from build123d import *

# Parameters (mm, degrees)
SKETCH1_R           = 4.1
BOSS_EXTRUDE1_DEPTH = 4.5
SKETCH2_W           = 4
SKETCH2_H           = 26
BOSS_EXTRUDE2_DEPTH = 58
SKETCH3_W           = 5
SKETCH3_H           = 26
BOSS_EXTRUDE3_DEPTH = 38
CUT_EXTRUDE1_START  = -5
CUT_EXTRUDE1_DEPTH  = 3
SKETCH6_R           = 4.2
CUT_EXTRUDE2_DEPTH  = 10
FILLET1_R           = 12
CUT_EXTRUDE4_DEPTH  = 74
SKETCH8_R           = 1.599994812
SKETCH8_R_2         = 1.6
SKETCH8_R_3         = 1.599991008
CUT_EXTRUDE5_DEPTH  = 8.5
CUT_EXTRUDE6_DEPTH  = 2
SKETCH10_W          = 7
SKETCH10_H          = 2.5
CUT_EXTRUDE7_DEPTH  = 114


with BuildPart() as part:
    # Sketch1 → Boss-Extrude1 (new body)
    with BuildSketch(Plane.XY):
        with BuildLine():
            Line((58.8, 13), (93.910980652, 13))
            Line((93.910980652, 13), (93.910980652, -13))
            Line((93.910980652, -13), (58.8, -13))
            ThreePointArc((58.8, -13), (45.8, 0), (58.8, 13))
        make_face()
        with Locations((58.8, 0)):
            Circle(SKETCH1_R, mode=Mode.SUBTRACT)
    extrude(amount=BOSS_EXTRUDE1_DEPTH)

    # Sketch2 → Boss-Extrude2 (add)
    with BuildSketch(Plane.XY.offset(4.5)):
        with Locations((91.910980652, 0)):
            Rectangle(SKETCH2_W, SKETCH2_H)
    extrude(amount=BOSS_EXTRUDE2_DEPTH)

    # Sketch3 → Boss-Extrude3 (add)
    with BuildSketch(Plane.ZY.offset(-89.910980652)):
        with Locations((60, 0)):
            Rectangle(SKETCH3_W, SKETCH3_H)
    extrude(amount=BOSS_EXTRUDE3_DEPTH)

    # Sketch5 → Cut-Extrude1 (cut)
    with BuildSketch(Plane.XY.offset(62.5).offset(CUT_EXTRUDE1_START)):
        with BuildLine():
            Line((75.8, 1.8), (59.925839282, 3.994369276))
            ThreePointArc((59.925839282, 3.994369276), (54.65, 6.2252e-05), (59.925719446, -3.99440305))
            Line((59.925719446, -3.99440305), (75.8, -1.799997977))
            ThreePointArc((75.8, -1.799997977), (77.599998989, 1.011e-06), (75.8, 1.8))
        make_face()
    extrude(amount=CUT_EXTRUDE1_DEPTH, mode=Mode.SUBTRACT)

    # Sketch6 → Cut-Extrude2 (cut)
    with BuildSketch(Plane.XY.offset(62.5)):
        with Locations((58.8, 0)):
            Circle(SKETCH6_R)
    extrude(amount=-CUT_EXTRUDE2_DEPTH, mode=Mode.SUBTRACT)

    # Fillet1
    fillet1_edges = [part.edges().sort_by_distance(p)[0] for p in [
        (51.910980652, 13, 60),
        (51.910980652, -13, 60),
    ]]
    fillet(fillet1_edges, radius=FILLET1_R)

    # Sketch7 → Cut-Extrude4 (cut)
    with BuildSketch(Plane(origin=(0, 0, 0), x_dir=(-1, 0, 0), z_dir=(0, 0, -1))):
        Polygon((-56.262443614, -3.220373827), (-56.262443614, 3.220373827), (-53.042069787, 0), align=None)
    extrude(amount=-CUT_EXTRUDE4_DEPTH, mode=Mode.SUBTRACT)

    # Sketch8 → Cut-Extrude5 (cut)
    with BuildSketch(Plane(origin=(93.910980652, 0, 0), x_dir=(0, 0, -1), z_dir=(1, 0, 0))):
        with Locations((-53.458782271, -8.985219923)):
            Circle(SKETCH8_R)
        with Locations((-53.458782271, 9)):
            Circle(SKETCH8_R_2)
        with Locations((-33.458782271, 9)):
            Circle(SKETCH8_R_2)
        with Locations((-33.458782271, -8.985219923)):
            Circle(SKETCH8_R_3)
    extrude(amount=-CUT_EXTRUDE5_DEPTH, mode=Mode.SUBTRACT)

    # Sketch9 → Cut-Extrude6 (cut)
    with BuildSketch(Plane.ZY.offset(-89.910980652)):
        Polygon((30.587828745, -7.37661001), (30.630208458, -10.667233653), (33.501161984, -12.275843566), (36.329735796, -10.593829837), (36.287356083, -7.303206194), (33.416402558, -5.69459628), align=None)
        Polygon((30.584160019, 10.602044603), (30.63405982, 7.311526406), (33.508682072, 5.709481802), (36.333404522, 7.397955397), (36.283504721, 10.688473594), (33.408882469, 12.290518198), align=None)
        Polygon((50.589182836, -7.374195689), (50.62879464, -10.664853815), (53.498394075, -12.27587805), (56.328381705, -10.596244158), (56.288769901, -7.305586031), (53.419170466, -5.694561797), align=None)
        Polygon((50.692796157, 7.216934993), (53.619968806, 5.713053256), (56.38595492, 7.496118262), (56.224768384, 10.783065007), (53.297595735, 12.286946744), (50.531609621, 10.503881738), align=None)
    extrude(amount=-CUT_EXTRUDE6_DEPTH, mode=Mode.SUBTRACT)

    # Sketch10 → Cut-Extrude7 (cut)
    with BuildSketch(Plane(origin=(0, 0, 0), x_dir=(-1, 0, 0), z_dir=(0, 0, -1))):
        with Locations((-84.62488512, 9.639193317)):
            Rectangle(SKETCH10_W, SKETCH10_H)
    extrude(amount=-CUT_EXTRUDE7_DEPTH, mode=Mode.SUBTRACT)


solid = part.part
Build history of the part. All positions in model axes, mm. A direction names the side the tool comes from. Give positions to 0.01 mm unless a question says otherwise; leave off trailing zeros. Loops run counter-clockwise (first coordinate to the right, second up) from the corner with the lowest first, then second, coordinate; pieces in that order, holes last. Notation, with made-up numbers: (-26, -39) - (4, -39) arc R23 cw to (4, -31) - close; hole circle Ø1 at (78, 24.25). An arc over 180 degrees is marked (long way). Write item = value, one per line. Start each with the question number.
1) Probe probe 1 along Z at (x, y) = (75.5, 6.25); probe 2 along X at (y, z) = (2.5, 55.5); probe 3 along Z at (x, y) = (52.5, -10). List the from-to ranges inside material, lowest first. Write a range as from..to.
2) Drop flat-ended pins along their axis: pin 1 Ø6.5 at (y, z) = (-7.5, 32.5) entering from -X; pin 2 Ø3 at (y, z) = (9, 53.46) entering from +X; pin 3 Ø3.5 at (y, z) = (-8.99, 53.46) entering from -X. Give the stop position or say it passes through.
3) Pull direction Y, two halves, no side cores. Call faces 4 (the cylindrical face through (55.52, -9.58, 60.04)), 5 (the flat face through (68, 0, 4.5)), 6 (the cylindrical face through (55.84, -2.98, 60.59)), 7 (the flat face through (90.9, -6.51, 34.87)): +Y half, -Y half, draft (parallel to the pull), parting line (faces both ways), or undercut.
4) Band-saw the part on A-A on z = 38. Give the cut face in (x, y), plus the area to 3 significant figures.
5) Tool access for faces 1 (the flat face through (90.897, -11.447, 34.896)), 2 (the flat face through (54.1, -1.06, 59.96)), 3 (the flat face through (68.12, 2.86, 58.98)): list every direction of +Z, -Z, +X, -X, +Y, -Y with a clear straight run to the whole face (end or side of a thin tool).
Final values:
q1.probe_1 = 0..4.5, 57.5..62.5
q1.probe_2 = 89.91..93.91
q1.probe_3 = 0..4.5
q2.pin_1 = 89.91
q2.pin_2 = through
q2.pin_3 = 91.91
q3.face_4 = -Y half
q3.face_5 = draft
q3.face_6 = undercut
q3.face_7 = undercut
q4.outline = (89.91, -13) - (93.91, -13) - (93.91, 13) - (89.91, 13) - close
q4.area = 104 mm²
q5.face_1 = -X
q5.face_2 = +Z, -Z
q5.face_3 = none
